Check sheet for the modelled part. Datum: model origin and axes. Units: mm. Coordinates: 2 decimals unless noted, no trailing zeros. Order: outer loops, then holes, each group sorted by start corner. A loop starts at its lowest first (then second) coordinate and runs counter-clockwise, first axis right, second up.
from build123d import *

# Parameters (mm, degrees)
SKETCH_2_R          = 2.5
SKETCH_2_R_2        = 4
SKETCH_2_R_3        = 2
EXTRUDE_11_DEPTH    = 3
SKETCH_2_16_R       = 4
SKETCH_2_16_R_2     = 2
EXTRUDE_12_DEPTH    = 0.5
SKETCH_2_17_R       = 2
EXTRUDE_13_DEPTH    = 12.5
FILLET_1_R          = 0.3
CUT_EXTRUDE_1_REACH = 52.966
SKETCH_3_R          = 1.5


with BuildPart() as part:
    # Sketch 2 → Extrude 11 (new body)
    # profile 1 of 7: a face of its own
    with BuildSketch(Plane.XY):
        Polygon((-41.985987982, 15.322651266), (-41.985987982, 21.467672234), (-25.900833035, 21.467672234), (-21.525354797, 25.843150472), (-14.576398582, 25.843150472), (-9.421808725, 23.655411353), (34.384238258, 23.655411353), (40.290588771, 21.148605879), (40.290588771, -26.048068749), (-41.985987982, -26.048068749), (-41.985987982, -12.123358681), (-33.943410509, -12.123358681), (-33.943410509, 11.301362529), (-37.964699246, 11.301362529), align=None)
        with Locations((9.574246485, 7.73050044)):
            Circle(SKETCH_2_R, mode=Mode.SUBTRACT)
        with Locations((-8.153758739, -18.910029411)):
            Circle(SKETCH_2_R, mode=Mode.SUBTRACT)
        with Locations((24.574246485, 17.73050044)):
            Circle(SKETCH_2_R_2, mode=Mode.SUBTRACT)
        with Locations((-29.162107176, 7.874269984)):
            Circle(SKETCH_2_R_2, mode=Mode.SUBTRACT)
        with Locations((-17.847699606, 19.897540861)):
            Circle(SKETCH_2_R, mode=Mode.SUBTRACT)
        with BuildLine():
            Line((24.695702599, -6.26949956), (30.574246485, -6.26949956))
            ThreePointArc((30.574246485, -6.26949956), (31.281353266, -5.976606341), (31.574246485, -5.26949956))
            Line((31.574246485, -5.26949956), (31.574246485, 0.609044326))
            ThreePointArc((31.574246485, 0.609044326), (31.228514311, 1.365307251), (30.430379263, 1.598641326))
            ThreePointArc((30.430379263, 1.598641326), (25.952143977, -0.647397052), (23.706105599, -5.125632338))
            ThreePointArc((23.706105599, -5.125632338), (23.939439675, -5.923767386), (24.695702599, -6.26949956))
        make_face(mode=Mode.SUBTRACT)
    # profile 2 of 7: a face of its own
    with BuildSketch(Plane.XY):
        with Locations((-29.162107176, 7.874269984)):
            Circle(SKETCH_2_R_2)
        with Locations((-29.162107176, 7.874269984)):
            Circle(SKETCH_2_R_3, mode=Mode.SUBTRACT)
    # profile 3 of 7: a face of its own
    with BuildSketch(Plane.XY):
        with Locations((-29.162107176, 7.874269984)):
            Circle(SKETCH_2_R_3)
    # profile 4 of 7: a face of its own
    with BuildSketch(Plane.XY):
        with Locations((24.574246485, 17.73050044)):
            Circle(SKETCH_2_R_2)
        with Locations((24.574246485, 17.73050044)):
            Circle(SKETCH_2_R_3, mode=Mode.SUBTRACT)
    # profile 5 of 7: a face of its own
    with BuildSketch(Plane.XY):
        with Locations((24.574246485, 17.73050044)):
            Circle(SKETCH_2_R_3)
    # profile 6 of 7: a face of its own
    with BuildSketch(Plane.XY):
        with BuildLine():
            ThreePointArc((24.695702599, -6.26949956), (23.939439675, -5.923767386), (23.706105599, -5.125632338))
            ThreePointArc((23.706105599, -5.125632338), (25.952143977, -0.647397052), (30.430379263, 1.598641326))
            ThreePointArc((30.430379263, 1.598641326), (31.228514311, 1.365307251), (31.574246485, 0.609044326))
            Line((31.574246485, 0.609044326), (31.574246485, -5.26949956))
            ThreePointArc((31.574246485, -5.26949956), (31.281353266, -5.976606341), (30.574246485, -6.26949956))
            Line((30.574246485, -6.26949956), (24.695702599, -6.26949956))
        make_face()
        with Locations((28.616748621, -3.312001696)):
            Circle(SKETCH_2_R_3, mode=Mode.SUBTRACT)
    # profile 7 of 7: a face of its own
    with BuildSketch(Plane.XY):
        with Locations((28.616748621, -3.312001696)):
            Circle(SKETCH_2_R_3)
    extrude(amount=EXTRUDE_11_DEPTH)

    # Sketch 2_16 → Extrude 12 (add)
    # profile 1 of 3: a face of its own
    with BuildSketch(Plane.XY):
        with Locations((-29.162107176, 7.874269984)):
            Circle(SKETCH_2_16_R)
        with Locations((-29.162107176, 7.874269984)):
            Circle(SKETCH_2_16_R_2, mode=Mode.SUBTRACT)
    # profile 2 of 3: a face of its own
    with BuildSketch(Plane.XY):
        with Locations((24.574246485, 17.73050044)):
            Circle(SKETCH_2_16_R)
        with Locations((24.574246485, 17.73050044)):
            Circle(SKETCH_2_16_R_2, mode=Mode.SUBTRACT)
    # profile 3 of 3: a face of its own
    with BuildSketch(Plane.XY):
        with BuildLine():
            ThreePointArc((24.695702599, -6.26949956), (23.939439675, -5.923767386), (23.706105599, -5.125632338))
            ThreePointArc((23.706105599, -5.125632338), (25.952143977, -0.647397052), (30.430379263, 1.598641326))
            ThreePointArc((30.430379263, 1.598641326), (31.228514311, 1.365307251), (31.574246485, 0.609044326))
            Line((31.574246485, 0.609044326), (31.574246485, -5.26949956))
            ThreePointArc((31.574246485, -5.26949956), (31.281353266, -5.976606341), (30.574246485, -6.26949956))
            Line((30.574246485, -6.26949956), (24.695702599, -6.26949956))
        make_face()
        with Locations((28.616748621, -3.312001696)):
            Circle(SKETCH_2_16_R_2, mode=Mode.SUBTRACT)
    extrude(amount=-EXTRUDE_12_DEPTH)

    # Sketch 2_17 → Extrude 13 (add)
    with BuildSketch(Plane.XY):
        with Locations((28.616748621, -3.312001696)):
            Circle(SKETCH_2_17_R)
        with Locations((24.574246485, 17.73050044)):
            Circle(SKETCH_2_17_R)
        with Locations((-29.162107176, 7.874269984)):
            Circle(SKETCH_2_17_R)
    extrude(amount=-EXTRUDE_13_DEPTH)

    # Fillet 1
    fillet_1_edges = [part.edges().sort_by_distance(p)[0] for p in [
        (26.616748621, -3.312001696, -12.5),
        (22.574246485, 17.73050044, -12.5),
        (-31.162107176, 7.874269984, -12.5),
    ]]
    fillet(fillet_1_edges, radius=FILLET_1_R)

    # Sketch 3 → Cut-Extrude 1 (cut, up to next)
    with BuildSketch(Plane(origin=(0, 0, 0), x_dir=(-1, 0, 0), z_dir=(0, 0, -1)), mode=Mode.PRIVATE) as cut_extrude_1_sk1:
        with Locations((-36.290588771, -19.088068749)):
            Circle(SKETCH_3_R)
    cut_extrude_1_tool1 = extrude(cut_extrude_1_sk1.sketch, amount=-CUT_EXTRUDE_1_REACH, mode=Mode.PRIVATE) & part.part
    # Sketch 3 → Cut-Extrude 1 (cut, up to next)
    with BuildSketch(Plane(origin=(0, 0, 0), x_dir=(-1, 0, 0), z_dir=(0, 0, -1)), mode=Mode.PRIVATE) as cut_extrude_1_sk2:
        with Locations((-30.290588771, -19.088068749)):
            Circle(SKETCH_3_R)
    cut_extrude_1_tool2 = extrude(cut_extrude_1_sk2.sketch, amount=-CUT_EXTRUDE_1_REACH, mode=Mode.PRIVATE) & part.part
    # Sketch 3 → Cut-Extrude 1 (cut, up to next)
    with BuildSketch(Plane(origin=(0, 0, 0), x_dir=(-1, 0, 0), z_dir=(0, 0, -1)), mode=Mode.PRIVATE) as cut_extrude_1_sk3:
        with Locations((31.985987982, -19.088068749)):
            Circle(SKETCH_3_R)
    cut_extrude_1_tool3 = extrude(cut_extrude_1_sk3.sketch, amount=-CUT_EXTRUDE_1_REACH, mode=Mode.PRIVATE) & part.part
    # Sketch 3 → Cut-Extrude 1 (cut, up to next)
    with BuildSketch(Plane(origin=(0, 0, 0), x_dir=(-1, 0, 0), z_dir=(0, 0, -1)), mode=Mode.PRIVATE) as cut_extrude_1_sk4:
        with Locations((37.985987982, -19.088068749)):
            Circle(SKETCH_3_R)
    cut_extrude_1_tool4 = extrude(cut_extrude_1_sk4.sketch, amount=-CUT_EXTRUDE_1_REACH, mode=Mode.PRIVATE) & part.part
    add(cut_extrude_1_tool1.solids().sort_by_distance((36.290589, -19.088069, 0))[0], mode=Mode.SUBTRACT)
    add(cut_extrude_1_tool2.solids().sort_by_distance((30.290589, -19.088069, 0))[0], mode=Mode.SUBTRACT)
    add(cut_extrude_1_tool3.solids().sort_by_distance((-31.985988, -19.088069, 0))[0], mode=Mode.SUBTRACT)
    add(cut_extrude_1_tool4.solids().sort_by_distance((-37.985988, -19.088069, 0))[0], mode=Mode.SUBTRACT)


solid = part.part
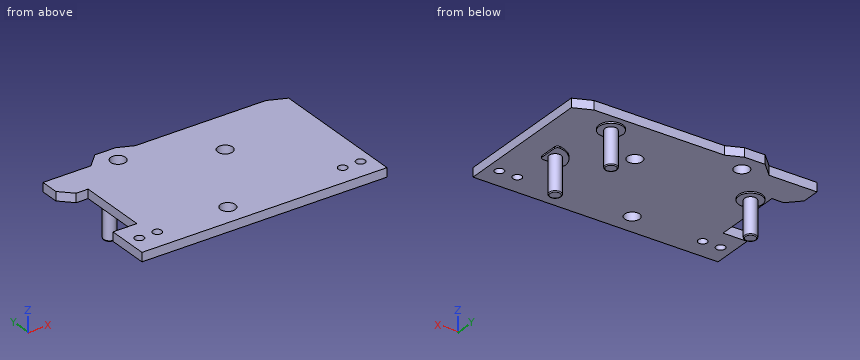
(1) Thickness scan on probe 1 along X at (y, z) = (-7.5, 2.25); probe 2 along Z at (x, y) = (-5.5, 17); probe 3 along Y at (x, z) = (23.5, -1.25). Record the ranges inside material, lowest first.
Filled in:
probe 1: x = -33.94 to 40.29
probe 2: z = 0 to 3
probe 3: y = 16.04 to 19.42
(2) Cross-section at A-A (x = -17.5). Enter the section's corners in (y, z).
Filled in:
outline: (-26.05, 0) - (17.42, 0) - (17.42, 3) - (-26.05, 3) - close; (22.37, 0) - (25.84, 0) - (25.84, 3) - (22.37, 3) - close
(3) Cross-section at C-C (y = -14.5). Enter the section's corners in (x, z).
Filled in:
outline: (-41.99, 0) - (40.29, 0) - (40.29, 3) - (-41.99, 3) - close
(4) Go/stop test with flat-tipped pins: P1, Ø1.5, axis at x = 10, z = 1.5, coming from the +Y side; P2, Ø5, axis at x = -23.5, y = -13.5, coming from the -Z side; P3, Ø2.5, axis at x = -36.5, z = 2, coming from the +Y side. Record where each tip stops, or that it passes through.
Filled in:
P1: stops at y = 23.66
P2: stops at z = 0
P3: stops at y = 21.47
(5) Cross-section at D-D (z = -5.75). Enter the section's corners in (x, y).
Filled in:
outline: circle Ø4 at (-29.16, 7.87); circle Ø4 at (24.57, 17.73); circle Ø4 at (28.62, -3.31)
(6) Cross-section at B-B (x = -2). Enter the section's corners in (y, z).
Filled in:
outline: (-26.05, 0) - (23.66, 0) - (23.66, 3) - (-26.05, 3) - close
